The model under review builds one solid part; all positions refer to its coordinate system, in mm. A direction names the side the tool comes from. Coordinates: 2 decimals unless noted, no trailing zeros. Write each loop counter-clockwise with the first axis right and the second up, starting at its lowest first coordinate (ties: lowest second). Pieces come first, ordered by that corner, then holes. Notation, with made-up numbers: (28.5, 3.5) - (67.5, 3.5) arc R17 ccw to (67.5, 36.5) - close; hole circle Ø6 at (11, 50.5). An arc over 180 degrees is marked (long way). Answer as CSV lines item,"result". Start each with the question number.
```python
from build123d import *

# Parameters (mm, degrees)
BOSS_EXTRUDE1_DEPTH     = 600
CUT_EXTRUDE1_DEPTH      = 600
CUT_EXTRUDE1_DEPTH_BACK = 600


with BuildPart() as part:
    # Sketch1 → Boss-Extrude1 (new body)
    with BuildSketch(Plane(origin=(0, 0, 0), x_dir=(0, 0, -1), z_dir=(1, 0, 0))):
        Polygon((30, 150), (30, 30), (570, 30), (570, 150), (600, 150), (600, 0), (0, 0), (0, 150), align=None)
    extrude(amount=BOSS_EXTRUDE1_DEPTH)

    # Sketch4 → Cut-Extrude1 (cut, two sides)
    with BuildSketch(Plane(origin=(0, 0, -30), x_dir=(-1, 0, 0), z_dir=(0, 0, -1))) as cut_extrude1_sk:
        Polygon((-600, 30), (-514.410107884, 150), (-600, 150), align=None)
    extrude(amount=CUT_EXTRUDE1_DEPTH, mode=Mode.SUBTRACT)
    extrude(cut_extrude1_sk.sketch, amount=-CUT_EXTRUDE1_DEPTH_BACK, mode=Mode.SUBTRACT)


solid = part.part
```
(1) The part is to be moulded in two halves that separate along Z. For faces 1 (the flat face through (296, 76, -600)), 2 (the flat face through (296, 30, -296)), 3 (the flat face through (557.804, 89.16, -584.79)), 4 (the flat face through (296, 91, -30)), say which applies: released by +Z, released by -Z, zero draft, split by the parting line, or undercut.
(2) For faces 5 (the flat face through (296, 89, -570)), 6 (the flat face through (254, 150, -585)), list the 3-axis set-ups (+Z, -Z, +X, -X, +Y, -Y) from which the entire face can be reached by the end or side of a thin tool; tool diameter is ignored.
(3) Add section C-C on y = 85. Give the boundary of the cut face in (x, z).
(4) Add section B-B on x = 83.5. Give the boundary of the cut face in (y, z).
(5) Add section D-D on z = -143. Give the boundary of the cut face in (x, y).
(6) Add section A-A on y = 121. Give the boundary of the cut face in (x, z), then the cut area to 3 significant figures.
(7) Wall thickness on line 1 (Z direction, x = 59.5, y = 90); line 2 (Y direction, x = 216.5, z = -569.5): over which ranges is each line inside the solid? List them lowest first.
(8) For pin 1 (1.5 mm diameter, centred on x = 519, z = -91, fed in from +Y), flat-tipped, find the tip position at first contact; note if it passes through.
Reported:
1,face 1,"released by -Z"
1,face 2,"undercut"
1,face 3,"zero draft"
1,face 4,"undercut"
2,face 5,"+X, -X, +Y"
2,face 6,"+Z, -Z, +X, -X, +Y"
3,outline,"(0, -600) - (560.77, -600) - (560.77, -570) - (0, -570) - close; (0, -30) - (560.77, -30) - (560.77, 0) - (0, 0) - close"
4,outline,"(0, -600) - (150, -600) - (150, -570) - (30, -570) - (30, -30) - (150, -30) - (150, 0) - (0, 0) - close"
5,outline,"(0, 0) - (600, 0) - (600, 30) - (0, 30) - close"
6,outline,"(0, -600) - (535.09, -600) - (535.09, -570) - (0, -570) - close; (0, -30) - (535.09, -30) - (535.09, 0) - (0, 0) - close"
6,area,"32,100 mm²"
7,line 1,"-600 to -570, -30 to 0"
7,line 2,"0 to 30"
8,pin 1,"y = 30"
